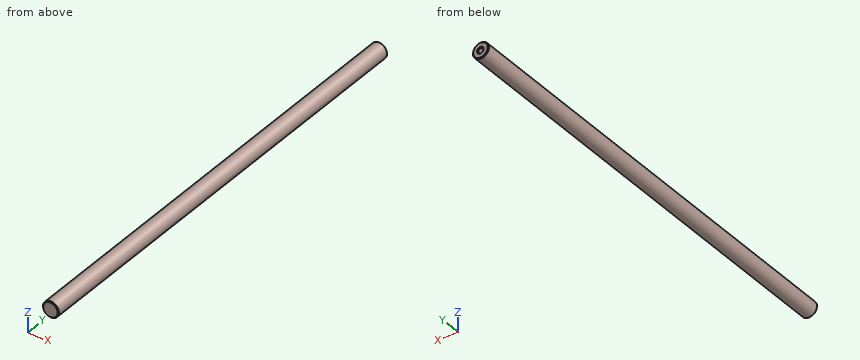
Autodesk Inventor part; units mm, degrees
ref_plane "YZ Plane" through (0, 0, 0) normal (1, 0, 0) x (0, 1, 0)
ref_plane "XZ Plane" through (0, 0, 0) normal (0, 1, 0) x (-1, 0, 0)
ref_plane "XY Plane" through (0, 0, 0) normal (0, 0, 1) x (1, 0, 0)
sketch "Sketch1" plane through (0, 0, 0) normal (0, 1, 0) x (-1, 0, 0)
  circle A0 centre (0, 0) radius 5
  dimension "d0" = 10
extrude "Extrusion1" add sketch "Sketch1" along normal blind 284
sketch "Sketch2" plane through (0, 284, 0) normal (0, 1, 0) x (1, 0, 0)
  point P0 (0, 0)
  point P1 (0, 0)
hole "Hole1" at (0, 284, 0) direction (0, -1, 0) diameter 3.242 depth 12 tip angle 118
chamfer "Chamfer1" distance 0.5 angle 45 3 edges at (0, 284, -1.621) (5, 284, 0) (5, 0, 0)
properties part number "CUT_ALU_10x284mm_Rod"
Check sheet for the modelled part. Datum: model origin and axes. Units: mm. Round coordinates to 2 decimals unless told otherwise and drop trailing zeros. Order: outer loops, then holes, each group sorted by start corner. A loop starts at its lowest first (then second) coordinate and runs counter-clockwise, first axis right, second up.
Q1. Scan lines: L1, parallel to Z at x = 0, y = 276; L2, parallel to Z at x = 0.5, y = 234. Record each from-to range of solid material in increasing order.
Filled sheet:
L1: z = -5 to -1.62, 1.62 to 5
L2: z = -4.97 to 4.97
Q2. Cross-section at A-A, the plane y = 19. Enter the section's corners in (x, z).
Filled sheet:
outline: circle Ø10 at (0, 0)
Q3. Depth check by flat-ended pin: P1, Ø2, axis at y = 214.5, z = -3, coming from the -X side; P2, Ø6, axis at y = 80.5, z = -0.5, coming from the +X side; P3, Ø3, axis at x = -3.5, y = 101.5, coming from the +Z side. Enter the tip coordinate at first touch or a pass-through.
Filled sheet:
P1: stops at x = -4.58
P2: stops at x = 5
P3: stops at z = 4.58
